from build123d import *

# Parameters (mm, degrees)
SKETCH1_W           = 8.5
SKETCH1_H           = 8.5
BOSS_EXTRUDE1_DEPTH = 5
SKETCH2_W           = 8.5
SKETCH2_H           = 8.5
BOSS_EXTRUDE2_DEPTH = 2
SKETCH3_R           = 1.5
CUT_EXTRUDE1_DEPTH  = 2
SKETCH4_W           = 54
SKETCH4_H           = 8.5
BOSS_EXTRUDE3_DEPTH = 3
SKETCH5_W           = 7
SKETCH5_H           = 8.5
BOSS_EXTRUDE4_DEPTH = 8.5
SKETCH8_R           = 1.5
BOSS_EXTRUDE5_DEPTH = 2.5
SKETCH9_R           = 1.5
BOSS_EXTRUDE6_DEPTH = 2.5
SKETCH10_W          = 8.5
SKETCH10_H          = 8.5
BOSS_EXTRUDE7_DEPTH = 1
CUT_EXTRUDE4_DEPTH  = 0.5
CUT_EXTRUDE5_DEPTH  = 0.5
SKETCH14_W          = 8.5
SKETCH14_H          = 8.5
BOSS_EXTRUDE8_DEPTH = 8
SKETCH15_W          = 8.5
SKETCH15_H          = 8.5
CUT_EXTRUDE6_DEPTH  = 1
SKETCH16_W          = 54
SKETCH16_H          = 3.5
CUT_EXTRUDE7_DEPTH  = 15
SKETCH17_W          = 5
SKETCH17_H          = 8.5
BOSS_EXTRUDE9_DEPTH = 7


with BuildPart() as part:
    # Sketch1 → Boss-Extrude1 (new body)
    with BuildSketch(Plane(origin=(0, 0, 0), x_dir=(0, 0, -1), z_dir=(1, 0, 0))):
        Rectangle(SKETCH1_W, SKETCH1_H)
        Polygon((1.705, 2.953146627), (-1.705, 2.953146627), (-3.41, 0), (-1.705, -2.953146627), (1.705, -2.953146627), (3.41, 0), align=None, mode=Mode.SUBTRACT)
    extrude(amount=BOSS_EXTRUDE1_DEPTH)

    # Sketch2 → Boss-Extrude2 (add)
    with BuildSketch(Plane.ZY):
        Rectangle(SKETCH2_W, SKETCH2_H)
    extrude(amount=BOSS_EXTRUDE2_DEPTH)

    # Sketch3 → Cut-Extrude1 (cut)
    with BuildSketch(Plane(origin=(0, 0, 0), x_dir=(0, 0, -1), z_dir=(1, 0, 0))):
        Circle(SKETCH3_R)
    extrude(amount=-CUT_EXTRUDE1_DEPTH, mode=Mode.SUBTRACT)

    # Sketch4 → Boss-Extrude3 (add)
    with BuildSketch(Plane.XZ.offset(4.25)):
        with Locations((25, 0)):
            Rectangle(SKETCH4_W, SKETCH4_H)
    extrude(amount=BOSS_EXTRUDE3_DEPTH)

    # Sketch5 → Boss-Extrude4 (add)
    with BuildSketch(Plane(origin=(0, -4.25, 0), x_dir=(1, 0, 0), z_dir=(0, 1, 0))):
        with Locations((48.5, 0)):
            Rectangle(SKETCH5_W, SKETCH5_H)
    extrude(amount=BOSS_EXTRUDE4_DEPTH)

    # Sketch8 → Boss-Extrude5 (add)
    with BuildSketch(Plane(origin=(0, 0, 0), x_dir=(0, 0, -1), z_dir=(1, 0, 0))):
        Polygon((-1.705, 2.953146627), (-3.41, 0), (-1.705, -2.953146627), (1.705, -2.953146627), (3.41, 0), (1.705, 2.953146627), align=None)
        Circle(SKETCH8_R, mode=Mode.SUBTRACT)
    extrude(amount=BOSS_EXTRUDE5_DEPTH)

    # Sketch9 → Boss-Extrude6 (add)
    with BuildSketch(Plane.ZY.offset(-50)):
        Polygon((3.41, 0), (1.705, 2.953146627), (-1.705, 2.953146627), (-3.41, 0), (-1.705, -2.953146627), (1.705, -2.953146627), align=None)
        with Locations(Location((0, 0, 0), (0, 0, 180))):
            Circle(SKETCH9_R, mode=Mode.SUBTRACT)
    extrude(amount=BOSS_EXTRUDE6_DEPTH)

    # Sketch10 → Boss-Extrude7 (add)
    with BuildSketch(Plane(origin=(5, 0, 0), x_dir=(0, 0, -1), z_dir=(1, 0, 0))):
        Rectangle(SKETCH10_W, SKETCH10_H)
        Polygon((3.41, 0), (1.705, 2.953146627), (-1.705, 2.953146627), (-3.41, 0), (-1.705, -2.953146627), (1.705, -2.953146627), align=None, mode=Mode.SUBTRACT)
    extrude(amount=BOSS_EXTRUDE7_DEPTH)

    # Sketch12 → Cut-Extrude4 (cut)
    with BuildSketch(Plane(origin=(2.5, 0, 0), x_dir=(0, 0, -1), z_dir=(1, 0, 0))):
        Polygon((1.705, -2.953146627), (3.41, 0), (1.705, 2.953146627), (-1.705, 2.953146627), (-3.41, 0), (-1.705, -2.953146627), align=None)
    extrude(amount=-CUT_EXTRUDE4_DEPTH, mode=Mode.SUBTRACT)

    # Sketch13 → Cut-Extrude5 (cut)
    with BuildSketch(Plane.ZY.offset(-47.5)):
        Polygon((1.705, 2.953146627), (-1.705, 2.953146627), (-3.41, 0), (-1.705, -2.953146627), (1.705, -2.953146627), (3.41, 0), align=None)
    extrude(amount=-CUT_EXTRUDE5_DEPTH, mode=Mode.SUBTRACT)

    # Sketch14 → Boss-Extrude8 (add)
    with BuildSketch(Plane(origin=(6, 0, 0), x_dir=(0, 0, -1), z_dir=(1, 0, 0))):
        Rectangle(SKETCH14_W, SKETCH14_H)
    extrude(amount=-BOSS_EXTRUDE8_DEPTH)

    # Sketch15 → Cut-Extrude6 (cut)
    with BuildSketch(Plane(origin=(6, 0, 0), x_dir=(0, 0, -1), z_dir=(1, 0, 0))):
        Rectangle(SKETCH15_W, SKETCH15_H)
    extrude(amount=-CUT_EXTRUDE6_DEPTH, mode=Mode.SUBTRACT)

    # Sketch16 → Cut-Extrude7 (cut)
    with BuildSketch(Plane(origin=(0, 4.25, 0), x_dir=(1, 0, 0), z_dir=(0, 1, 0))):
        with Locations((25, 2.5)):
            Rectangle(SKETCH16_W, SKETCH16_H)
    extrude(amount=-CUT_EXTRUDE7_DEPTH, mode=Mode.SUBTRACT)

    # Sketch17 → Boss-Extrude9 (add)
    with BuildSketch(Plane.ZY.offset(-45)):
        with Locations((1.75, 0)):
            Rectangle(SKETCH17_W, SKETCH17_H)
    extrude(amount=-BOSS_EXTRUDE9_DEPTH)


solid = part.part
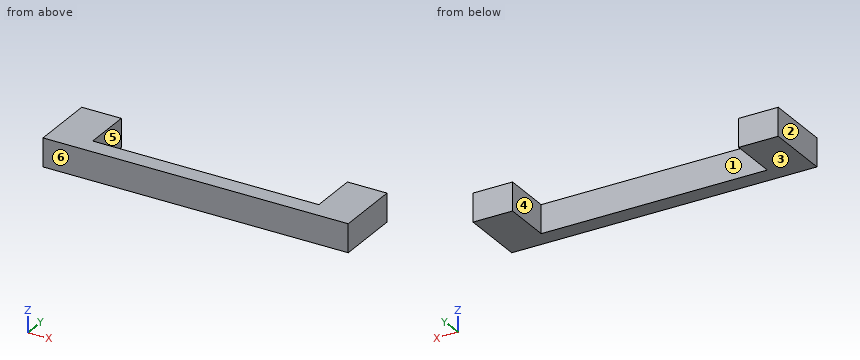
Part model, mm, in its own coordinate system. Face numbers are marked on the shaded views. A direction names the side the tool comes from. Coordinates: 2 decimals unless noted, no trailing zeros. Loops run counter-clockwise (first coordinate to the right, second up) from the corner with the lowest first, then second, coordinate; pieces in that order, holes last. Notation, with made-up numbers: M 65,-16.75 L 114,-16.75 A23 ccw 114,-8.75 Z; hole C -35.5,-29 d3. An arc over 180 degrees is marked long. Use a Markdown table: item, result. Add a question column.
Q1. Which spindle directions (+Z, -Z, +X, -X, +Y, -Y) get a long thin tool onto all of the face, cutting with end or side? Do the marked faces 5 and 6. Say none if no direction does.
Q2. Cut at A-A (y = 3.75). Write the cut outline in (x, z).
Q3. Cut at C-C (x = 38). Write the cut outline in (y, z), and give its area (3 significant figures).
Q4. Probe L1, parallel to X at y = -1.75, z = -0.4; L2, parallel to Y at x = 39.5, z = 3.55. List the from-to ranges inside material, lowest first.
Q5. Pin check, flat tips, straight feed: P1, Ø3, axis at x = 32, z = 2.5, coming from the +Y side; P2, Ø5, axis at x = 17, y = -2.5, coming from the -Z side. Stop position of each tip, or through.
Q6. Mould opens along X. For the marked faces 1, 2, 3 and 4 say: +X half, -X half, draft (parallel to the pull), parting line (faces both ways), or undercut.
Q7. Cut at B-B (z = 0.2). Write the cut outline in (x, y), and give its area (3 significant figures).
Worked out:
| question | item | result |
|---|---|---|
| 1 | face 5 | +Z, -Z, +Y |
| 1 | face 6 | +Z, -Z, +X, -X, -Y |
| 2 | outline | M -2,-0.75 L 5,-0.75 L 5,4.25 L -2,4.25 Z; M 45,-0.75 L 52,-0.75 L 52,4.25 L 45,4.25 Z |
| 3 | outline | M -7.25,-0.75 L -4.25,-0.75 L -4.25,4.25 L -7.25,4.25 Z |
| 3 | area | 15.0 mm2 |
| 4 | L1 | x = -2 to 5, 45 to 52 |
| 4 | L2 | y = -7.25 to -4.25 |
| 5 | P1 | stops at y = -4.25 |
| 5 | P2 | stops at z = -0.75 |
| 6 | face 1 | undercut |
| 6 | face 2 | -X half |
| 6 | face 3 | draft |
| 6 | face 4 | undercut |
| 7 | outline | M -2,-7.25 L 52,-7.25 L 52,4.25 L 45,4.25 L 45,-4.25 L 5,-4.25 L 5,4.25 L -2,4.25 Z |
| 7 | area | 281 mm2 |
